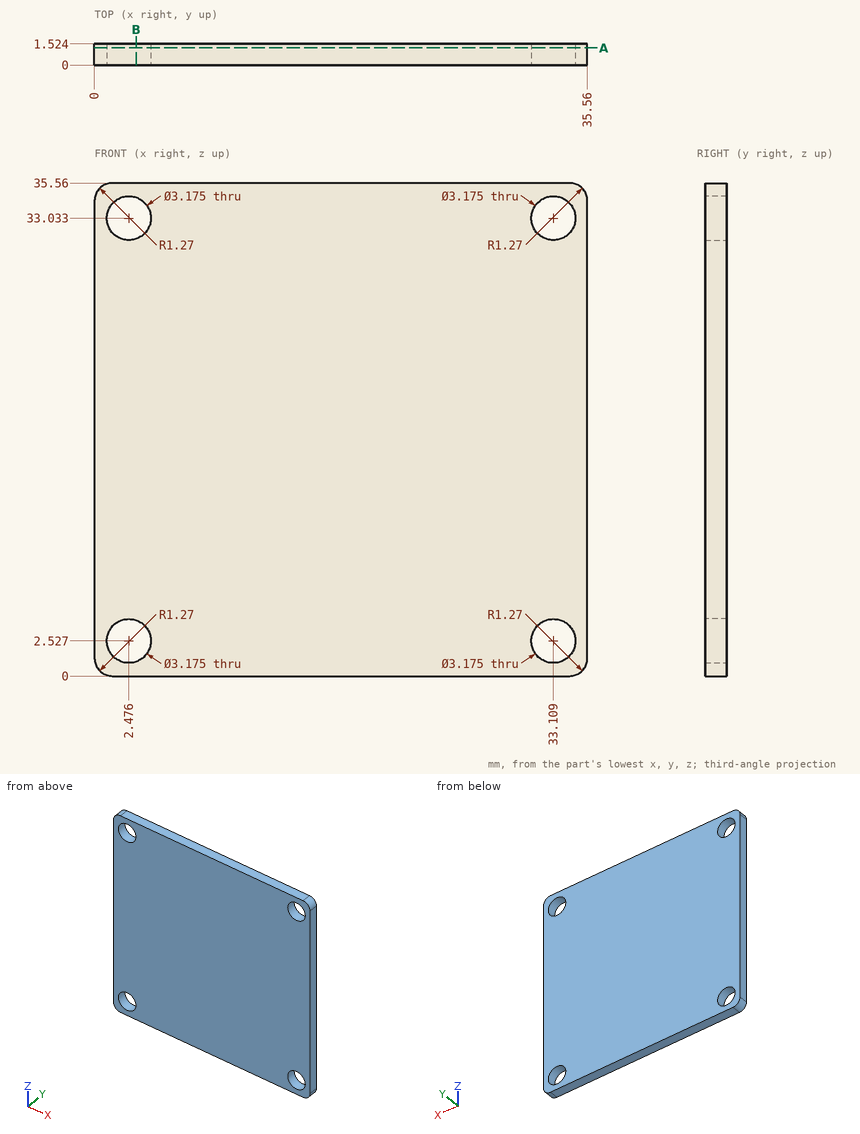
Design review of the part shown in the three views and the two pictorial views. Dimensions are in mm from the part's minimum x, y and z. Give positions to 0.01 mm unless a question says otherwise; leave off trailing zeros. Order: outer loops, then holes, each group sorted by start corner. A loop starts at its lowest first (then second) coordinate and runs counter-clockwise, first axis right, second up. Notation, with made-up numbers: M -13.75,35.25 L 38.25,35.25 A29 ccw 38.25,69.25 Z; hole C -34.75,-11.5 d6. An arc over 180 degrees is marked long. Answer in a Markdown table with one row per item. Add a question column.
(1) Wall thickness on probe 1 along X at (y, z) = (1.25, 33) (1 decimal); probe 2 along X at (y, z) = (0.4, 32) (1 decimal); probe 3 along Z at (x, y) = (32, 0.75) (1 decimal): over which ranges is each line inside the solid? List them lowest first. Write a range as [from, to].
(2) Consider section A-A on y = 1.25. State the section outline as (x, z) points (1 decimal).
(3) Consider section B-B on x = 3. State the section outline as (y, z) points (1 decimal).
(4) For pin 1 (1.9 mm diameter, centred on x = 2.48, z = 33.03, fed in from -Y), flat-tipped, find the tip position at first contact; note if it passes through.
Evaluation:
| question | item | result |
|---|---|---|
| 1 | probe 1 | x = [0, 0.9], [4.1, 31.5], [34.7, 35.6] |
| 1 | probe 2 | x = [0, 1.3], [3.7, 31.9], [34.3, 35.6] |
| 1 | probe 3 | z = [0, 1.4], [3.7, 31.9], [34.2, 35.6] |
| 2 | outline | M 0,1.3 A1.3 ccw 1.3,0 L 34.3,0 A1.3 ccw 35.6,1.3 L 35.6,34.3 A1.3 ccw 34.3,35.6 L 1.3,35.6 A1.3 ccw 0,34.3 Z; hole C 2.5,2.5 d3.2; hole C 2.5,33 d3.2; hole C 33.1,2.5 d3.2; hole C 33.1,33 d3.2 |
| 3 | outline | M 0,0 L 1.5,0 L 1.5,1 L 0,1 Z; M 0,4 L 1.5,4 L 1.5,31.5 L 0,31.5 Z; M 0,34.5 L 1.5,34.5 L 1.5,35.6 L 0,35.6 Z |
| 4 | pin 1 | passes through |
